The listing builds one solid part. Answer for the finished solid, in the listing's coordinates (mm). Face numbers are marked on the shaded views. A direction names the side the tool comes from. Round coordinates to 2 decimals unless told otherwise and drop trailing zeros. Loops run counter-clockwise (first coordinate to the right, second up) from the corner with the lowest first, then second, coordinate; pieces in that order, holes last. Notation, with made-up numbers: M 34,69 L 71,69 A28 ccw 71,87 Z; hole C -20.75,56.5 d10. An arc over 180 degrees is marked long. Answer as a JSON object with one key per item and string values.
```python
from build123d import *

# Parameters (mm, degrees)
CUT_EXTRUDE_5_DEPTH = 1.2


with BuildPart() as part:
    # 草图2 → 旋转1 (revolve)
    with BuildSketch(Plane.XY):
        with BuildLine():
            Line((0, 0), (0, 1.5))
            Line((0, 1.5), (-19.1, 1.5))
            Line((-19.1, 1.5), (-19.1, 1.05))
            Line((-19.1, 1.05), (-20, 1.05))
            Line((-20, 1.05), (-20, 2.8))
            Line((-20, 2.8), (-20.8, 2.8))
            ThreePointArc((-20.8, 2.8), (-21.971790212, 1.61245155), (-22.4, 0))
            Line((-22.4, 0), (0, 0))
        make_face()
    revolve(axis=Axis((0, 0, 0), (-1, 0, 0)))

    # 草图3 → 切除-拉伸5 (cut)
    with BuildSketch(Plane(origin=(-22.4, 0, 0), x_dir=(0, 0, -1), z_dir=(1, 0, 0))):
        with BuildLine():
            Line((0.375, 1.8), (-0.375, 1.8))
            Line((-0.375, 1.8), (-0.375, 0.675))
            ThreePointArc((-0.375, 0.675), (-0.462867966, 0.462867966), (-0.675, 0.375))
            Line((-0.675, 0.375), (-1.8, 0.375))
            Line((-1.8, 0.375), (-1.8, -0.375))
            Line((-1.8, -0.375), (-0.675, -0.375))
            ThreePointArc((-0.675, -0.375), (-0.462867966, -0.462867966), (-0.375, -0.675))
            Line((-0.375, -0.675), (-0.375, -1.8))
            Line((-0.375, -1.8), (0.375, -1.8))
            Line((0.375, -1.8), (0.375, -0.675))
            ThreePointArc((0.375, -0.675), (0.462867966, -0.462867966), (0.675, -0.375))
            Line((0.675, -0.375), (1.8, -0.375))
            Line((1.8, -0.375), (1.8, 0.375))
            Line((1.8, 0.375), (0.675, 0.375))
            ThreePointArc((0.675, 0.375), (0.462867966, 0.462867966), (0.375, 0.675))
            Line((0.375, 0.675), (0.375, 1.8))
        make_face()
    extrude(amount=CUT_EXTRUDE_5_DEPTH, mode=Mode.SUBTRACT)


solid = part.part
```
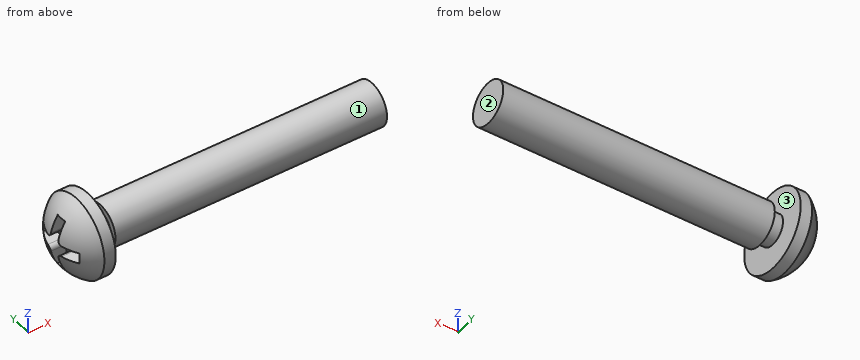
Item 1: The part is cut by section D-D (x = -4.5). Give the vertices of the cut face in (y, z), then the cut area to 3 significant figures.
Values follow:
{"outline": "C 0,0 d3", "area": "7.07 mm^2"}
Item 2: Flat-ended cylindrical pins translate along their axes: P1, Ø0.9, axis at x = -21.5, y = 1.5, coming from the -Z side; P2, Ø2.5, axis at y = 0.5, z = 0.5, coming from the -X side; P3, Ø1.5, axis at x = -17.5, z = 1.5, coming from the -Y side; P4, Ø0.6, axis at x = -21.5, z = -1.5, coming from the -Y side. Find the tip coordinate at first contact, or state that the pin passes through.
Values follow:
{"P1": "z = -2.26", "P2": "x = -22.33", "P3": "y = -1.3", "P4": "y = -2.09"}
Item 3: The part is cut by section C-C (z = 1.3). Give the vertices of the cut face in (x, y) (3 decimals).
Values follow:
{"outline": "M -22.105,-0.375 A2.979 ccw -20.8,-2.48 L -20,-2.48 L -20,2.48 L -20.8,2.48 A2.979 ccw -22.105,0.375 L -21.2,0.375 L -21.2,-0.375 Z; M -19.1,-0.748 L 0,-0.748 L 0,0.748 L -19.1,0.748 Z"}
Item 4: The part is cut by section A-A (y = 0). Give the vertices of the cut face in (x, z).
Values follow:
{"outline": "M -21.86,-1.8 A3.25 ccw -20.8,-2.8 L -20,-2.8 L -20,-1.05 L -19.1,-1.05 L -19.1,-1.5 L 0,-1.5 L 0,1.5 L -19.1,1.5 L -19.1,1.05 L -20,1.05 L -20,2.8 L -20.8,2.8 A3.25 ccw -21.86,1.8 L -21.2,1.8 L -21.2,-1.8 Z"}
Item 5: Straight lines are drawn through the part: line 1 (X direction, y = -0.1, z = 1.1); line 2 (Y direction, x = -7.5, z = -0.1); line 3 (X direction, y = -0.4, z = 0.2). For each, find the intervals that lie inside material, in ascending order.
Values follow:
{"line 1": "-21.2 to -20, -19.1 to 0", "line 2": "-1.5 to 1.5", "line 3": "-21.2 to 0"}
Item 6: Which of the six approach directions +Z, -Z, +X, -X, +Y, -Y give full straight-line access (tool end or side, diameter ignored) to the marked faces 1, 2 and 3?
Values follow:
{"face 1": "+X", "face 2": "+Z, -Z, +X, +Y, -Y", "face 3": "none"}
